from build123d import *

# Parameters (mm, degrees)
SKETCH1_R           = 1.25
SKETCH1_R_2         = 3
SKETCH1_R_3         = 2
SKETCH1_W           = 2
SKETCH1_H           = 5
BOSS_EXTRUDE1_DEPTH = 5


with BuildPart() as part:
    # Sketch1 → Boss-Extrude1 (new body)
    with BuildSketch(Plane.XY):
        with BuildLine():
            Line((-15.5, 55), (-15.5, 0))
            ThreePointArc((-15.5, 0), (0, -11.5), (15.5, 0))
            Line((15.5, 0), (15.5, 55))
            ThreePointArc((15.5, 55), (0, 66.5), (-15.5, 55))
        make_face()
        with Locations((0, 7)):
            Circle(SKETCH1_R, mode=Mode.SUBTRACT)
        with Locations((7, 0)):
            Circle(SKETCH1_R, mode=Mode.SUBTRACT)
        with Locations((0, -7)):
            Circle(SKETCH1_R, mode=Mode.SUBTRACT)
        with Locations((-7, 0)):
            Circle(SKETCH1_R, mode=Mode.SUBTRACT)
        with Locations((0, 20)):
            Circle(SKETCH1_R_2, mode=Mode.SUBTRACT)
        with Locations((2.5, 58)):
            Circle(SKETCH1_R_3, mode=Mode.SUBTRACT)
        with Locations((2.5, 43)):
            Circle(SKETCH1_R_3, mode=Mode.SUBTRACT)
        with Locations((-4.5, 50.5)):
            Circle(SKETCH1_R_3, mode=Mode.SUBTRACT)
        with Locations((11, 30.5)):
            Rectangle(SKETCH1_W, SKETCH1_H, mode=Mode.SUBTRACT)
    extrude(amount=BOSS_EXTRUDE1_DEPTH)


solid = part.part
For this review, take the finished solid that the model builds, in its own axes (mm). A direction names the side the tool comes from. Coordinates: 2 decimals unless noted, no trailing zeros. Write each loop counter-clockwise with the first axis right and the second up, starting at its lowest first coordinate (ties: lowest second). Pieces come first, ordered by that corner, then holes. Notation, with made-up numbers: (-39.75, -27.5) -> (-12.75, -27.5) arc R26 cw to (-12.75, 9.5) -> close; hole circle Ø6 at (-11, -39). An arc over 180 degrees is marked (long way). Write each question's results on one line, items separated by ' | '. Start each with the question number.
1) Consider section D-D (x = 2). Write out the cut boundary in (y, z), plus the area to 3 significant figures.
2) For faces 1 (the face through (11, 28, 2)), 2 (the face through (0, 28, 5)), list the 3-axis set-ups (+Z, -Z, +X, -X, +Y, -Y) from which the entire face can be reached by the end or side of a thin tool; tool diameter is ignored.
3) Insertion check: pin 1 (1.6 mm diameter, centred on x = 10.5, z = 2.5, fed in from -Y); pin 2 (2 mm diameter, centred on x = 11, z = 1.5, fed in from +Y). Each pin has a flat end and moves straight along its axis. Give the tip position at first contact, or say it passes through.
4) Consider section C-C (x = -4). Write out the cut boundary in (y, z).
5) The part is to be moulded in two halves that separate along Y. For faces 3 (the face through (10, 30, 2)), 4 (the face through (0.289, 66.497, 2.465)), 5 (the face through (0, 28, 0)), say which applies: +Y half, -Y half, draft (parallel to the pull), parting line (faces both ways), or undercut.
6) Consider section A-A (y = 20). Write out the cut boundary in (x, z).
7) Consider section B-B (z = 3.25). Give the number of separate pieces and of enclosed holes in the cut face, plus the area to 3 significant figures.
8) Wall thickness on L1, parallel to X at y = 21.5, z = 4.4; L2, parallel to Y at x = 2.5, z = 2.65; L3, parallel to X at y = 51, z = 0.6: over which ranges is each line inside the solid? List them lowest first. Write a range as [from, to].
Geometry says:
1) outline: (-11.38, 0) -> (17.76, 0) -> (17.76, 5) -> (-11.38, 5) -> close; (22.24, 0) -> (41.06, 0) -> (41.06, 5) -> (22.24, 5) -> close; (44.94, 0) -> (56.06, 0) -> (56.06, 5) -> (44.94, 5) -> close; (59.94, 0) -> (66.38, 0) -> (66.38, 5) -> (59.94, 5) -> close | area: 328 mm^2
2) face 1: +Z, -Z | face 2: +Z, +X, -X, +Y, -Y
3) pin 1: y = -8.27 | pin 2: y = 63.04
4) outline: (-11, 0) -> (48.56, 0) -> (48.56, 5) -> (-11, 5) -> close; (52.44, 0) -> (66, 0) -> (66, 5) -> (52.44, 5) -> close
5) face 3: undercut | face 4: +Y half | face 5: draft
6) outline: (-15.5, 0) -> (-3, 0) -> (-3, 5) -> (-15.5, 5) -> close; (3, 0) -> (15.5, 0) -> (15.5, 5) -> (3, 5) -> close
7) separate pieces: 1 | enclosed holes: 9 | area: 2,130 mm^2
8) L1: [-15.5, -2.6], [2.6, 15.5] | L2: [-11.31, 18.34], [21.66, 41], [45, 56], [60, 66.31] | L3: [-15.5, -6.44], [-2.56, 15.5]
